Autodesk Fusion 360 part; units mm, degrees
sketch "Sketch1" plane through (0, 0, 0) normal (0, 1, 0) x (1, 0, 0) in component "base_plate"
  line L0 (0, 0) -> (35, 0)
  line L1 (35, 0) -> (35, -20)
  line L2 (0, 0) -> (0, -20)
  line L3 (0, -20) -> (35, -20)
  dimension "d1" = 35
  dimension "d2" = 20
  dimension "d3" = 20
extrude "Extrude1" add sketch "Sketch1" along normal blind 5 in component "base_plate"
sketch "Sketch2" plane through (0, 0, 0) normal (0, -1, 0) x (1, 0, 0) in component "base_plate"
  line L0 (0, 20) -> (0, 0)
  line L1 (0, 0) -> (35, 0)
  line L2 (35, 0) -> (35, 20)
  line L3 (35, 20) -> (0, 20)
  line L4 (0, 10) -> (35, 10) construction
  line L5 (17.5, 20) -> (17.5, 0) construction
  circle A0 centre (7.6246, 10) radius 1
  circle A1 centre (26.0211, 10) radius 1
  dimension "d6" = 2
  dimension "d7" = 2
extrude "Extrude2" cut sketch "Sketch2" against normal blind 5 contours A0 | A1 in component "base_plate"
sketch "Sketch3" plane through (0, 0, 0) normal (0, -1, 0) x (1, 0, 0) in component "base_plate"
  circle A0 centre (7.6246, 10) radius 1
  circle A1 centre (26.0211, 10) radius 1
  line L0 (0, 20) -> (0, 0)
  line L1 (0, 0) -> (35, 0)
  line L2 (35, 0) -> (35, 20)
  line L3 (35, 20) -> (0, 20)
  line L4 (17.5, 20) -> (17.5, 0) construction
  circle A2 centre (17.5, 16.2296) radius 1
  circle A3 centre (17.5, 3.7004) radius 1
  dimension "d10" = 2
  dimension "d11" = 2
extrude "Extrude3" cut sketch "Sketch3" against normal blind 5 contours A2 | A3 in component "base_plate"
sketch "Sketch4" plane through (0, 0, 0) normal (0, -1, 0) x (1, 0, 0) in component "base_plate"
  circle A0 centre (17.5, 3.7004) radius 1
  circle A1 centre (17.5, 16.2296) radius 1
  circle A2 centre (7.6246, 10) radius 1
  circle A3 centre (26.0211, 10) radius 1
  line L0 (0, 20) -> (0, 0)
  line L1 (0, 0) -> (35, 0)
  line L2 (35, 0) -> (35, 20)
  line L3 (35, 20) -> (0, 20)
  line L4 (17.5, 20) -> (17.5, 0) construction
  circle A4 centre (17.5, 10) radius 11.5
extrude "Extrude4" cut sketch "Sketch4" against normal blind 3 contours A0 | A1 | A2 | A3 | L1 L3 A4 in component "base_plate"
component "base_plate" placed x (1, 0, 0) y (0, 1, 0) z (0, 0, 1) at (0, 0, 0)
Part model, mm, in its own coordinate system. A direction names the side the tool comes from. Coordinates: 2 decimals unless noted, no trailing zeros. Order: outer loops, then holes, each group sorted by start corner. A loop starts at its lowest first (then second) coordinate and runs counter-clockwise, first axis right, second up. Notation, with made-up numbers: (38, 16) - (78, 16) arc R19 cw to (78, 50) - close; hole circle Ø9 at (86, -24.75). An arc over 180 degrees is marked (long way). Use CSV: the item, a comma, the result in double quotes.
Item 1: Mould opens along Z. For faces 3 (the face through (17, 5, 10)), 4 (the face through (17, 4, 20)), 5 (the face through (7.49, 3.99, 10.99)), 6 (the face through (17, 4, 0)) say: +Z half, -Z half, draft (parallel to the pull), parting line (faces both ways), or undercut.
Solved:
face 3,"draft"
face 4,"+Z half"
face 5,"undercut"
face 6,"-Z half"
Item 2: Saw through at C-C on y = 1.85. Give the cut face in (x, z), and give its area (3 significant figures).
Solved:
outline,"(0, 0) - (11.82, 0) arc R11.5 cw to (11.82, 20) - (0, 20) - close; (23.18, 0) - (35, 0) - (35, 20) - (23.18, 20) arc R11.5 cw to start"
area,"308 mm²"
Item 3: Saw through at D-D on z = 14.5. Give the cut face in (x, y), and give its area (3 significant figures).
Solved:
outline,"(0, 0) - (6.92, 0) - (6.92, 3) - (28.08, 3) - (28.08, 0) - (35, 0) - (35, 5) - (0, 5) - close"
area,"112 mm²"
Item 4: Saw through at B-B on z = 10. Give the cut face in (x, y).
Solved:
outline,"(0, 0) - (6, 0) - (6, 3) - (6.62, 3) - (6.62, 5) - (0, 5) - close; (8.62, 3) - (25.02, 3) - (25.02, 5) - (8.62, 5) - close; (27.02, 3) - (29, 3) - (29, 0) - (35, 0) - (35, 5) - (27.02, 5) - close"
Item 5: Probe probe 1 along Z at (x, y) = (17.5, 4.4); probe 2 along Y at (x, z) = (13, 11); probe 3 along Z at (x, y) = (17, 3.1). List the from-to ranges inside material, lowest first.
Solved:
probe 1,"z = 0 to 2.7, 4.7 to 15.23, 17.23 to 20"
probe 2,"y = 3 to 5"
probe 3,"z = 0 to 2.83, 4.57 to 15.36, 17.1 to 20"
Item 6: Drop flat-ended pins along their axis: P1, Ø1.2, axis at x = 7.62, z = 10, coming from the -Y side; P2, Ø3, axis at x = 26.02, z = 10, coming from the -Y side. Give the stop position or say it passes through.
Solved:
P1,"passes through"
P2,"stops at y = 3"
Item 7: 3-axis set-ups, long thin cutter, end or side, ignore diameter. For faces 1 (the face through (17, 3, 10)), 2 (the face through (5, 0, 10)): which of +Z, -Z, +X, -X, +Y, -Y reach the whole face in a straight line?
Solved:
face 1,"-Y"
face 2,"+Z, -Z, +X, -X, -Y"
Item 8: Saw through at A-A on x = 17.5. Give the cut face in (y, z).
Solved:
outline,"(3, 0) - (5, 0) - (5, 2.7) - (3, 2.7) - close; (3, 4.7) - (5, 4.7) - (5, 15.23) - (3, 15.23) - close; (3, 17.23) - (5, 17.23) - (5, 20) - (3, 20) - close"
